Model file for the job. Use its own axes, mm. A direction names the side the tool comes from. Coordinates: 2 decimals unless noted, no trailing zeros. Write each loop counter-clockwise with the first axis right and the second up, starting at its lowest first coordinate (ties: lowest second). Pieces come first, ordered by that corner, then holes. Notation, with made-up numbers: (-35, -19) -> (-18, -19) arc R23 ccw to (-18, 6) -> close; hole circle Ø8 at (22, 20.25). An arc over 180 degrees is marked (long way). Answer as a JSON object with one key per item and string values. Group by question number.
Autodesk Inventor part; units mm, degrees
ref_plane "YZ Plane" through (0, 0, 0) normal (1, 0, 0) x (0, 1, 0)
ref_plane "XZ Plane" through (0, 0, 0) normal (0, 1, 0) x (-1, 0, 0)
ref_plane "XY Plane" through (0, 0, 0) normal (0, 0, 1) x (1, 0, 0)
sketch "Sketch1" plane through (0, 0, 0) normal (0, 1, 0) x (-1, 0, 0)
  line L0 (-10.16, 10.16) -> (10.16, 10.16)
  line L1 (10.16, 10.16) -> (10.16, -10.16)
  line L2 (10.16, -10.16) -> (-10.16, -10.16)
  line L3 (-10.16, -10.16) -> (-10.16, 10.16)
  circle A0 centre (0, 0) radius 8.255
  dimension "d0" = 20.32
  dimension "d1" = 20.32
  dimension "d2" = 10.16
  dimension "d3" = 10.16
  dimension "d4" = 16.51
extrude "Extrusion1" add sketch "Sketch1" along normal blind 12.7
sketch "Sketch2" plane through (10.16, 0, 10.16) normal (1, 0, 0) x (0, 0, -1)
  line L0 (1.778, 12.446) -> (2.921, 5.08)
  line L1 (2.921, 5.08) -> (17.399, 5.08)
  line L2 (17.399, 5.08) -> (18.542, 12.446)
  line L3 (18.542, 12.446) -> (1.778, 12.446)
  line L4 (20.32, 0) -> (0, 0)
  line L5 (20.32, 0) -> (20.32, 12.7)
  point P0 (10.16, 0)
  dimension "d7" = 16.764
  dimension "d8" = 14.478
  dimension "d9" = 7.366
  dimension "d10" = 5.08
  dimension "d11" = 2.921
extrude "Extrusion2" add sketch "Sketch2" along normal blind 12.7
sketch "Sketch3" plane through (10.16, 12.446, 8.382) normal (0, 1, 0) x (1, 0, 0)
  circle A0 centre (5.842, 8.382) radius 2.286
  line L0 (12.7, 16.764) -> (12.7, 0)
  point P0 (-10.16, 8.382)
  dimension "d14" = 4.572
  dimension "d15" = 6.858
extrude "Extrusion3" cut sketch "Sketch3" against normal blind 17.78
sketch "Sketch4" plane through (10.16, 12.446, 8.382) normal (0, 1, 0) x (1, 0, 0)
  circle A0 centre (5.842, 8.382) radius 2.286
  line L0 (0, 0) -> (0, 16.764)
  line L1 (0, 0) -> (12.7, 0)
  line L2 (12.7, 16.764) -> (12.7, 0)
  line L3 (0, 16.764) -> (12.7, 16.764)
  point P0 (-10.16, 8.382)
extrude "Extrusion4" add sketch "Sketch4" along normal up to surface (0.254 mm away)
properties part number "HopperFinal2"
(1) Cut at D-D on y = 11.5. List the corners of the cut face in (x, z) (3 decimals).
(2) Wall check: probe 1 along Z at (x, y) = (0, 10) (3 decimals); probe 2 along X at (y, z) = (11.75, 1.5); probe 3 along Y at (x, z) = (16, -6.5). Give the ranges that are in metal, low to high.
(3) 3-axis set-ups, long thin cutter, end or side, ignore diameter. For faces 1 (the face through (16.421, 8.815, 7.819)), 2 (the face through (18, 5.08, 2)), 3 (the face through (-10.16, 6, 0)): which of +Z, -Z, +X, -X, +Y, -Y reach the whole face in a straight line?
(4) Pull direction Z, two halves, no side cores. Call faces 4 (the face through (18.11, 8.84, -0.88)), 5 (the face through (10, 12.7, 0)), 6 (the face through (16.4, 8.7, -7.8)), 7 (the face through (-7.874, 6.261, -2.48)): released by +Z, released by -Z, zero draft, split by the parting line, or undercut.
(5) Pin check, flat tips, straight feed: pin 1 (6.5 mm diameter, centred on x = 18.5, z = -0.5, fed in from -Y); pin 2 (4 mm diameter, centred on x = 12, z = -0.5, fed in from -Y). Stop position of each tip, or through.
(6) Cut at C-C on z = -3.75. List the corners of the cut face in (x, y), plus the area to 3 significant figures.
(7) Cut at B-B on y = 1.5. List the corners of the cut face in (x, z) (3 decimals).
(8) Cut at A-A on x = 0. List the corners of the cut face in (y, z) (3 decimals), plus the area to 3 significant figures.
Results found:
{
 "1": {"outline": "(-10.16, -10.16) -> (10.16, -10.16) -> (10.16, -8.235) -> (22.86, -8.235) -> (22.86, 8.235) -> (10.16, 8.235) -> (10.16, 10.16) -> (-10.16, 10.16) -> close; hole circle Ø16.51 at (0, 0); hole circle Ø4.572 at (16.002, 0)"},
 "2": {"probe 1": "z = -10.16 to -8.255, 8.255 to 10.16", "probe 2": "x = -10.16 to -8.12, 8.12 to 14.28, 17.73 to 22.86", "probe 3": "y = 5.08 to 12.7"},
 "3": {"face 1": "+Z, +X, -Y", "face 2": "+Z, -Z, +X, -Y", "face 3": "+Z, -Z, -X, +Y, -Y"},
 "4": {"face 4": "undercut", "face 5": "zero draft", "face 6": "released by -Z", "face 7": "undercut"},
 "5": {"pin 1": "stops at y = 5.08", "pin 2": "stops at y = 0"},
 "6": {"outline": "(-10.16, 0) -> (-7.35, 0) -> (-7.35, 12.7) -> (-10.16, 12.7) -> close; (7.35, 0) -> (10.16, 0) -> (10.16, 5.08) -> (22.86, 5.08) -> (22.86, 12.7) -> (7.35, 12.7) -> close", "area": "168 mm²"},
 "7": {"outline": "(-10.16, -10.16) -> (10.16, -10.16) -> (10.16, 10.16) -> (-10.16, 10.16) -> close; hole circle Ø16.51 at (0, 0)"},
 "8": {"outline": "(0, -10.16) -> (12.7, -10.16) -> (12.7, -8.255) -> (0, -8.255) -> close; (0, 8.255) -> (12.7, 8.255) -> (12.7, 10.16) -> (0, 10.16) -> close", "area": "48.4 mm²"}
}
